Design review of the part built by this model. Coordinates are the model's own, in mm. A direction names the side the tool comes from. Give positions to 0.01 mm unless a question says otherwise; leave off trailing zeros. Loops run counter-clockwise (first coordinate to the right, second up) from the corner with the lowest first, then second, coordinate; pieces in that order, holes last. Notation, with made-up numbers: M 25,39 L 68,39 A12 ccw 68,51 Z; hole C 43,-10.75 d2. An arc over 180 degrees is marked long. Use CSV: the item, a comma, the result in double quotes.
from build123d import *

# Parameters (mm, degrees)
SKETCH1_R            = 2.5
BOSS_EXTRUDE1_DEPTH  = 27
SKETCH2_R            = 0.825
CUT_EXTRUDE1_DEPTH   = 5
FILLET1_R            = 0.5
FILLET1_OF_MIRROR1_R = 0.5


with BuildPart() as part:
    # Sketch1 → Boss-Extrude1 (new body)
    with BuildSketch(Plane(origin=(0, 0, 0), x_dir=(1, 0, 0), z_dir=(0, 1, 0))):
        with Locations(Location((0, 0, 0), (0, 0, 270))):
            Circle(SKETCH1_R)
    boss_extrude1 = extrude(amount=BOSS_EXTRUDE1_DEPTH)

    # Sketch2 → Cut-Extrude1 (cut)
    with BuildSketch(Plane(origin=(0, 27, 0), x_dir=(1, 0, 0), z_dir=(0, 1, 0))):
        with Locations(Location((0, 0, 0), (0, 0, 270))):
            Circle(SKETCH2_R)
    cut_extrude1 = extrude(amount=-CUT_EXTRUDE1_DEPTH, mode=Mode.SUBTRACT)

    # Fillet1
    fillet1_edges = [part.edges().sort_by_distance(p)[0] for p in [
        (0, 27, -2.5),
    ]]
    fillet(fillet1_edges, radius=FILLET1_R)

    # Mirror1: Boss-Extrude1, Cut-Extrude1 across plane
    add(boss_extrude1.mirror(Plane.ZX))
    add(cut_extrude1.mirror(Plane.ZX), mode=Mode.SUBTRACT)

    # Fillet1 of Mirror1
    fillet1_of_mirror1_edges = [part.edges().sort_by_distance(p)[0] for p in [
        (0, -27, -2.5),
    ]]
    fillet(fillet1_of_mirror1_edges, radius=FILLET1_OF_MIRROR1_R)


solid = part.part
(1) Wall thickness on line 1 along X through (y, z) = (23.45, 0) (3 decimals); line 2 along X through (y, z) = (-8, 1.5); line 3 along Y through (x, z) = (-2, -0.5): over which ranges is each line inside the solid? List them lowest first. Write a range as [from, to].
A:
line 1,"[-2.5, -0.825], [0.825, 2.5]"
line 2,"[-2, 2]"
line 3,"[-27, 27]"
(2) We need section C-C on y = 17.5. State the section outline as (x, z) points, then the cut area to 3 significant figures.
A:
outline,"C 0,0 d5"
area,"19.6 mm²"
(3) Machinability: for faces 5 (the flat face through (0, -27, 1)), 6 (the flat face through (0, -22, 0)), which of the approach directions +Z, -Z, +X, -X, +Y, -Y give a long, thin tool a straight path to every point of the face, cutting with its end or side? Answer none if there is none.
A:
face 5,"+Z, -Z, +X, -X, -Y"
face 6,"-Y"
(4) Clearance check with flat-ended pins moving along their axes: P1, Ø1.5, axis at y = 13.5, z = 1, coming from the +X side; P2, Ø1, axis at y = -15.5, z = -1.5, coming from the -X side; P3, Ø1.5, axis at x = 0, z = 0, coming from the -Y side. State where each tip first meets the part, or that it passes through.
A:
P1,"x = 2.49"
P2,"x = -2.29"
P3,"y = -22"
(5) We need section B-B on x = 0. State the section outline as (y, z) points (3 decimals), then the cut area to 3 significant figures.
A:
outline,"M -27,-2 A0.5 ccw -26.5,-2.5 L 26.5,-2.5 A0.5 ccw 27,-2 L 27,-0.825 L 22,-0.825 L 22,0.825 L 27,0.825 L 27,2 A0.5 ccw 26.5,2.5 L -26.5,2.5 A0.5 ccw -27,2 L -27,0.825 L -22,0.825 L -22,-0.825 L -27,-0.825 Z"
area,"253 mm²"
(6) The part is to be moulded in two halves that separate along Z. For faces 1 (the flat face through (0, 27, 1)), 2 (the cylindrical face through (-0.502, 24.535, -0.655)), 3 (the flat face through (0, 22, 0)), 4 (the cylindrical face through (-2.44, 0.37, -0.54)), say which applies: released by +Z, released by -Z, zero draft, split by the parting line, or undercut.
A:
face 1,"zero draft"
face 2,"undercut"
face 3,"undercut"
face 4,"split by the parting line"
(7) We need section A-A on z = 0. State the section outline as (x, y) points (3 decimals).
A:
outline,"M -2.5,-26.5 A0.5 ccw -2,-27 L -0.825,-27 L -0.825,-22 L 0.825,-22 L 0.825,-27 L 2,-27 A0.5 ccw 2.5,-26.5 L 2.5,26.5 A0.5 ccw 2,27 L 0.825,27 L 0.825,22 L -0.825,22 L -0.825,27 L -2,27 A0.5 ccw -2.5,26.5 Z"
